For this review, take the finished solid that the model builds, in its own axes (mm). A direction names the side the tool comes from. Round coordinates to 2 decimals unless told otherwise and drop trailing zeros. Loops run counter-clockwise (first coordinate to the right, second up) from the corner with the lowest first, then second, coordinate; pieces in that order, holes last.
1) Take a section at C-C (z = -38). State the section outline as (x, y) points.
2) Take a section at B-B (x = -75). State the section outline as (y, z) points, then the cut area to 3 significant figures.
3) Wall thickness on L1, parallel to Z at x = -75, y = 6.25; L2, parallel to X at y = 5.5, z = -61.5; L3, parallel to Z at x = -27.5, y = 8.5: over which ranges is each line inside the solid? List them lowest first.
4) Tool access review of faces 1 (the flat face through (-3, 19, -34)), 2 (the flat face through (-46, 7, -16.5)), 3 (the flat face through (-26, 25, -67)): name each direction out of +Z, -Z, +X, -X, +Y, -Y from which nothing blocks a thin tool from reaching the whole face with its end or side.
5) Take a section at D-D (y = 16.5). State the section outline as (x, z) points.
6) Insertion check: pin 1 (1.5 mm diameter, centred on y = 26.5, z = -67, fed in from +X); pin 2 (10 mm diameter, centred on x = -54.5, z = -33, fed in from +Y); pin 3 (2 mm diameter, centred on x = -17, z = -59, fed in from +Y). Each pin has a flat end and moves straight along its axis. Give the tip position at first contact, or say it passes through.
7) Take a section at A-A (y = 6.5). State the section outline as (x, z) points.
Autodesk Inventor part; units mm, degrees
ref_plane "YZ Plane" through (0, 0, 0) normal (1, 0, 0) x (0, 1, 0)
ref_plane "XZ Plane" through (0, 0, 0) normal (0, 1, 0) x (-1, 0, 0)
ref_plane "XY Plane" through (0, 0, 0) normal (0, 0, 1) x (1, 0, 0)
sketch "Sketch1" plane through (0, 0, 0) normal (0, 1, 0) x (-1, 0, 0)
  line L0 (0, 0) -> (91, 0)
  line L1 (91, 0) -> (91, -68)
  line L2 (91, -68) -> (0, -68)
  line L3 (0, -68) -> (0, 0)
  line L4 (88, -3) -> (3, -3)
  line L5 (3, -3) -> (3, -65)
  line L6 (3, -65) -> (88, -65)
  line L7 (88, -65) -> (88, -3)
  dimension "d0" = 91
  dimension "d1" = 68
  dimension "d2" = 62
  dimension "d3" = 85
  dimension "d4" = 3
  dimension "d5" = 3
extrude "Extrusion1" add sketch "Sketch1" along normal blind 29 contours L0 L1 L2 L3 | L7 L6 L5 L4
sketch "Sketch2" plane through (0, 29, 0) normal (0, 1, 0) x (1, 0, 0)
  line L0 (-88, 16.5) -> (-3, 16.5)
  line L1 (-3, 16.5) -> (-3, 51.5)
  line L2 (-3, 51.5) -> (-88, 51.5)
  line L3 (-88, 51.5) -> (-88, 16.5)
  line L4 (-91, 68) -> (-91, 0)
  line L5 (0, 68) -> (-91, 68)
  point P0 (0, 0)
  dimension "d8" = 85
  dimension "d9" = 35
  dimension "d10" = 3
  dimension "d11" = 16.5
extrude "Extrusion2" cut sketch "Sketch2" against normal blind 26
sketch "Sketch3" plane through (0, 29, 0) normal (0, 1, 0) x (1, 0, 0)
  line L0 (-88, 3) -> (-3, 3)
  line L1 (-3, 3) -> (-3, 65)
  line L2 (-3, 65) -> (-88, 65)
  line L3 (-88, 65) -> (-88, 3)
  line L4 (-91, 68) -> (-91, 0)
  line L5 (0, 68) -> (-91, 68)
  point P0 (0, 0)
  point P1 (-45.5, 68)
  dimension "d14" = 62
  dimension "d15" = 85
  dimension "d16" = 3
  dimension "d17" = 3
extrude "Extrusion3" cut sketch "Sketch3" against normal blind 16
sketch "Sketch4" plane through (0, 0, -68) normal (0, 0, -1) x (-1, 0, 0)
  line L0 (88, 29) -> (3, 29)
  line L1 (10, 29) -> (26, 29)
  line L2 (26, 29) -> (26, 20)
  line L3 (26, 20) -> (10, 20)
  line L4 (10, 20) -> (10, 29)
  line L5 (0, 0) -> (0, 29)
  point P0 (26, 29)
  dimension "d20" = 16
  dimension "d21" = 9
  dimension "d22" = 10
extrude "Extrusion4" cut sketch "Sketch4" against normal blind 4
sketch "Sketch5" plane through (0, 13, 0) normal (0, 1, 0) x (1, 0, 0)
  circle A0 centre (-75, 7.5) radius 0.95
  line L0 (-88, 3) -> (-88, 65)
  line L1 (-3, 3) -> (-88, 3)
  circle A1 centre (-10.5, 61.5) radius 0.95
  line L2 (-88, 65) -> (-26, 65)
  line L3 (-3, 65) -> (-3, 3)
  point P0 (0, 0)
  dimension "d25" = 1.9
  dimension "d26" = 13
  dimension "d27" = 4.5
  dimension "d28" = 1.9
  dimension "d29" = 3.5
  dimension "d30" = 7.5
extrude "Extrusion5" cut sketch "Sketch5" against normal blind 10
fillet "Fillet1" radius 2 8 edges at (0, 14.5, -68) (0, 14.5, 0) (0, 0, -34) (-45.5, 0, -68) (-91, 14.5, -68) (-91, 14.5, 0) (-91, 0, -34) (-45.5, 0, 0)
sketch "Sketch6" plane through (-88, 3, -16.5) normal (1, 0, 0) x (0, 0, -1)
  line L0 (0, 0) -> (15, 0)
  line L1 (15, 0) -> (15, 27)
  line L2 (15, 27) -> (0, 27)
  line L3 (0, 27) -> (0, 0)
  point P0 (-16.5, -3)
  dimension "d34" = 15
  dimension "d35" = 27
extrude "Extrusion6" cut sketch "Sketch6" against normal blind 10
fillet "Fillet2" radius 1 5 edges at (-88, 16, -31.5) (-91, 16, -31.5) (-91, 16, -16.5) (-88, 21, -16.5) (-91, 3, -24)
properties part number "Glove Case"
Response:
1. outline: (-91, 2) arc R2 ccw to (-89, 0) - (-2, 0) arc R2 ccw to (0, 2) - (0, 29) - (-3, 29) - (-3, 3) - (-88, 3) - (-88, 29) - (-91, 29) - close
2. outline: (0, -66) arc R2 ccw to (2, -68) - (29, -68) - (29, -65) - (13, -65) - (13, -51.5) - (3, -51.5) - (3, -16.5) - (13, -16.5) - (13, -8.45) - (3, -8.45) - (3, -6.55) - (13, -6.55) - (13, -3) - (29, -3) - (29, 0) - (2, 0) arc R2 ccw to (0, -2) - close
2. area: 609 mm2
3. L1: z = -68 to -51.5, -16.5 to -8.45, -6.55 to 0
3. L2: x = -91 to -11.45, -9.55 to 0
3. L3: z = -68 to -51.5, -16.5 to 0
4. face 1: +Y
4. face 2: -X, +Y
4. face 3: -Z, +Y
5. outline: (-91, -66) arc R2 ccw to (-89, -68) - (-2, -68) arc R2 ccw to (0, -66) - (0, -2) arc R2 ccw to (-2, 0) - (-89, 0) arc R2 ccw to (-91, -2) - (-91, -15.5) arc R1 ccw to (-90, -16.5) - (-89, -16.5) arc R1 ccw to (-88, -15.5) - (-88, -3) - (-3, -3) - (-3, -65) - (-88, -65) - (-88, -32.5) arc R1 ccw to (-89, -31.5) - (-90, -31.5) arc R1 ccw to (-91, -32.5) - close
6. pin 1: stops at x = -0.02
6. pin 2: stops at y = 3
6. pin 3: stops at y = 13
7. outline: (-91, -66) arc R2 ccw to (-89, -68) - (-2, -68) arc R2 ccw to (0, -66) - (0, -2) arc R2 ccw to (-2, 0) - (-89, 0) arc R2 ccw to (-91, -2) - (-91, -15.5) arc R1 ccw to (-90, -16.5) - (-3, -16.5) - (-3, -51.5) - (-88, -51.5) - (-88, -32.5) arc R1 ccw to (-89, -31.5) - (-90, -31.5) arc R1 ccw to (-91, -32.5) - close; hole circle Ø1.9 at (-75, -7.5); hole circle Ø1.9 at (-10.5, -61.5)
